Autodesk Inventor part; units mm, degrees
ref_plane "YZ Plane" through (0, 0, 0) normal (1, 0, 0) x (0, 1, 0)
ref_plane "XZ Plane" through (0, 0, 0) normal (0, 1, 0) x (-1, 0, 0)
ref_plane "XY Plane" through (0, 0, 0) normal (0, 0, 1) x (1, 0, 0)
sketch "Sketch4" plane through (0, 0, 0) normal (0, 1, 0) x (-1, 0, 0)
  line L0 (0, 0) -> (0, -12.6)
  line L1 (0, -12.6) -> (20, -12.6)
  line L2 (20, -12.6) -> (0, -12.6)
  line L3 (0, -12.6) -> (0, -15.6)
  line L4 (0, -15.6) -> (20, -15.6)
  line L5 (20, -15.6) -> (20, -12.6)
  line L6 (0, 0) -> (-12.9904, 7.5)
  line L7 (0, 0) -> (15, 0) construction
  line L8 (-12.9904, 7.5) -> (0, 0)
  line L9 (0, 0) -> (-1.5, -2.5981)
  line L10 (-1.5, -2.5981) -> (-14.4904, 4.9019)
  line L11 (-14.4904, 4.9019) -> (-12.9904, 7.5)
  line L12 (0, 0) -> (0, -15.6)
  line L13 (0, -15.6) -> (-3, -15.6)
  line L14 (-3, -15.6) -> (-3, 0)
  line L15 (-3, 0) -> (0, 0)
  dimension "d16" = 12.6
  dimension "d17" = 20
  dimension "d18" = 3
  dimension "d19" = 15
  dimension "d20" = 150
  dimension "d21" = 3
  dimension "d24" = 3
extrude "Extrusion5" add sketch "Sketch4" along normal blind 20
sketch "Sketch5" plane through (3, 0, -15.6) normal (0, 0, -1) x (-1, 0, 0)
  line L0 (3, 0) -> (23, 0)
  line L1 (13, 0) -> (13, 10)
  circle A0 centre (13, 10) radius 2.75
  dimension "d27" = 10
  dimension "d28" = 5.5
extrude "Extrusion6" cut sketch "Sketch5" against normal blind 3
sketch "Sketch6" plane through (3, 0, -1.7321) normal (0.5, 0, -0.866) x (-0.866, 0, -0.5)
  line L0 (0, 0) -> (0, 20)
  line L1 (0, 10) -> (-7, 10)
  circle A0 centre (-7, 10) radius 2.75
  point P0 (1.7321, 0)
  dimension "d31" = 7
  dimension "d32" = 5.5
extrude "Extrusion7" cut sketch "Sketch6" against normal blind 3
fillet "Fillet1" radius 5 2 edges at (3, 10, -1.7321) (3, 10, -15.6)
properties part number "Acrylic_angle_bracket"
Source: CAD feature listing. Evaluate the final solid. Frame: model axes, mm. A direction names the side the tool comes from. Give positions to 0.01 mm unless a question says otherwise; leave off trailing zeros. Write each loop counter-clockwise with the first axis right and the second up, starting at its lowest first coordinate (ties: lowest second). Pieces come first, ordered by that corner, then holes. Notation, with made-up numbers: (8, -19.5) - (35, -19.5) arc R26 ccw to (35, 17.5) - close; hole circle Ø11 at (4, 60.5). An arc over 180 degrees is marked (long way). One line per item, written item: value. Start each with the question number.
Q1. Set-up query: faces 1 (the face through (-20, 10, -14)), 2 (the face through (0, 10, -6)), 3 (the face through (3, 10, -8)). Return all of +Z, -Z, +X, -X, +Y, -Y with unobstructed straight access to the full face (end or side cutting, diameter ignored); none if empty.
Q2. Material intervals for probe 1 along Y at (x, z) = (-10, -14.2); probe 2 along Z at (x, y) = (-10.5, 2.5); probe 3 along X at (y, z) = (10, -14.7), sorted ascending. Write a range as from..to.
Q3. Section query C-C, the plane z = -8. Return the cut outline in (x, y), then the cut area to 3 significant figures.
Q4. Draft query along X for faces 4 (the face through (7.04, 12.32, 2.31)), 5 (the face through (3.65, 10.14, -2.15)), 6 (the face through (-11.48, 12.32, -14.12)), 7 (the face through (-12.1, 7.6, -12.6)). Return one class per face: +X half, -X half, draft (parallel to the pull), parting line (faces both ways), or undercut.
Q5. Section query D-D, the plane y = 10. Return the cut outline in (x, z), then the cut area to 3 significant figures.
Q6. Section query A-A, the plane x = -10. Return the cut outline in (y, z), then the cut area to 3 significant figures.
Q7. Section query B-B, the plane y = 12. Return the cut outline in (x, z).
Q8. First-contact query: pin 1 Ø3 at (y, z) = (6.5, -6.5) entering from +X; pin 2 Ø6 at (x, y) = (4.5, 2) entering from -Z; pin 3 Ø4.5 at (x, y) = (-10, 10) entering from -Z; pin 4 Ø6 at (x, y) = (-12.5, 14) entering from +Z. Flat tips, straight axial feed; report the tip coordinate or a pass-through.
Answer:
1. face 1: +Z, -Z, -X, +Y, -Y
1. face 2: +Z, -X, +Y, -Y
1. face 3: -Z, +X, +Y, -Y
2. probe 1: y = 0..7.25, 12.75..20
2. probe 2: z = -15.6..-12.6
2. probe 3: x = -20..-12.75, -7.25..0.86
3. outline: (0, 0) - (3, 0) - (3, 20) - (0, 20) - close
3. area: 60.0 mm2
4. face 4: undercut
4. face 5: +X half
4. face 6: undercut
4. face 7: draft
5. outline: (-20, -15.6) - (-12.75, -15.6) - (-12.75, -12.6) - (-20, -12.6) - close; (-7.25, -15.6) - (-2, -15.6) arc R5 ccw to (3, -10.6) - (3, -4.62) arc R5 cw to (5.5, -0.29) - (6.68, 0.39) - (5.18, 2.99) - (0, 0) - (0, -12.6) - (-7.25, -12.6) - close; (9.94, 5.74) - (11.44, 3.14) - (14.49, 4.9) - (12.99, 7.5) - close
5. area: 110 mm2
6. outline: (0, -15.6) - (7.25, -15.6) - (7.25, -12.6) - (0, -12.6) - close; (12.75, -15.6) - (20, -15.6) - (20, -12.6) - (12.75, -12.6) - close
6. area: 43.5 mm2
7. outline: (-20, -15.6) - (-11.89, -15.6) - (-11.89, -12.6) - (-20, -12.6) - close; (-8.11, -15.6) - (-2, -15.6) arc R5 ccw to (3, -10.6) - (3, -4.62) arc R5 cw to (5.5, -0.29) - (7.43, 0.82) - (5.93, 3.42) - (0, 0) - (0, -12.6) - (-8.11, -12.6) - close; (9.2, 5.31) - (10.7, 2.71) - (14.49, 4.9) - (12.99, 7.5) - close
8. pin 1: stops at x = 3
8. pin 2: stops at z = -14.17
8. pin 3: passes through
8. pin 4: stops at z = -12.6
